from build123d import *

# Parameters (mm, degrees)
SKETCH1_W           = 40
SKETCH1_H           = 40
BOSS_EXTRUDE1_DEPTH = 1000
SKETCH2_R           = 3.4
SKETCH2_W           = 6.95
SKETCH2_H           = 6.75
SKETCH2_W_2         = 6.75
SKETCH2_H_2         = 6.95
CUT_EXTRUDE1_DEPTH  = 1002.598722044
FILLET1_R           = 4.5


with BuildPart() as part:
    # Sketch1 → Boss-Extrude1 (new body)
    with BuildSketch(Plane(origin=(0, 0, 0), x_dir=(1, 0, 0), z_dir=(0, 1, 0))):
        with Locations((20, 20)):
            Rectangle(SKETCH1_W, SKETCH1_H)
    extrude(amount=BOSS_EXTRUDE1_DEPTH)

    # Sketch2 → Cut-Extrude1 (cut, through all)
    with BuildSketch(Plane(origin=(0, 1000, 0), x_dir=(1, 0, 0), z_dir=(0, 1, 0))):
        with Locations(Location((20, 20, 0), (0, 0, 270))):
            Circle(SKETCH2_R)
        Polygon((30.25, 31.75), (24, 25.5), (16, 25.5), (9.75, 31.75), (9.75, 38.2), (13.6, 38.2), (13.6, 35.75), (15.9, 35.75), (15.9, 40), (24.1, 40), (24.1, 35.75), (26.4, 35.75), (26.4, 38.2), (30.25, 38.2), align=None)
        Polygon((31.75, 9.75), (25.5, 16), (25.5, 24), (31.75, 30.25), (38.2, 30.25), (38.2, 26.4), (35.75, 26.4), (35.75, 24.1), (40, 24.1), (40, 15.9), (35.75, 15.9), (35.75, 13.6), (38.2, 13.6), (38.2, 9.75), align=None)
        with Locations((4.975, 35.125)):
            Rectangle(SKETCH2_W, SKETCH2_H)
        with Locations((35.125, 35.025)):
            Rectangle(SKETCH2_W_2, SKETCH2_H_2)
        Polygon((9.75, 8.25), (16, 14.5), (24, 14.5), (30.25, 8.25), (30.25, 1.8), (26.4, 1.8), (26.4, 4.25), (24.1, 4.25), (24.1, 0), (15.9, 0), (15.9, 4.25), (13.6, 4.25), (13.6, 1.8), (9.75, 1.8), align=None)
        with Locations((35.025, 4.875)):
            Rectangle(SKETCH2_W, SKETCH2_H)
        Polygon((8.25, 30.25), (14.5, 24), (14.5, 16), (8.25, 9.75), (1.8, 9.75), (1.8, 13.6), (4.25, 13.6), (4.25, 15.9), (0, 15.9), (0, 24.1), (4.25, 24.1), (4.25, 26.4), (1.8, 26.4), (1.8, 30.25), align=None)
        with Locations((4.875, 4.975)):
            Rectangle(SKETCH2_W_2, SKETCH2_H_2)
    extrude(amount=-CUT_EXTRUDE1_DEPTH, mode=Mode.SUBTRACT)

    # Fillet1
    fillet1_edges = [part.edges().sort_by_distance(p)[0] for p in [
        (38.5, 500, -38.5),
        (1.5, 500, -1.5),
        (38.5, 500, -1.5),
        (0, 500, -40),
        (40, 500, -40),
        (40, 500, 0),
        (0, 500, 0),
        (1.5, 500, -38.5),
    ]]
    fillet(fillet1_edges, radius=FILLET1_R)


solid = part.part
Build history of the part. All positions in model axes, mm. Give positions to 0.01 mm unless a question says otherwise; leave off trailing zeros. Use one line per item in the form item = value. Start each with the question number.
1. Drop flat-ended pins along their axis: pin 1 Ø1.2 at (x, y) = (2.5, 645.5) entering from +Z; pin 2 Ø0.7 at (y, z) = (302.5, -3) entering from +X; pin 3 Ø1.2 at (y, z) = (602.5, -37) entering from -X. Give the stop position or say it passes through.
2. Probe line 1 (Z direction, x = 4, y = 150.5); line 2 (Z direction, x = 4.5, y = 606); line 3 (X direction, y = 648, z = -7.5). List the from-to ranges inside material, lowest first. Write a range as [from, to].
3. Band-saw the part on A-A on y = 324.5. Count the separate pieces of the cut face and the enclosed holes in it, plus the area to 3 significant figures.
Conclusion:
q1.pin_1 = -0.22
q1.pin_2 = 39.85
q1.pin_3 = 0.09
q2.line_1 = [-39.97, -38.03], [-31.75, -30.25], [-26.4, -24.1], [-15.9, -13.6], [-9.75, -8.45], [-1.97, -0.03]
q2.line_2 = [-40, -38.24], [-31.75, -30.25], [-9.75, -8.45], [-1.76, 0]
q2.line_3 = [0, 1.5], [8.25, 9.75], [30.25, 31.55], [38.5, 40]
q3.separate_pieces = 1
q3.enclosed_holes = 5
q3.area = 477 mm²
